```python
from build123d import *

# Parameters (mm, degrees)
FILLET1_R          = 1
FILLET2_R          = 3
CHAMFER1_SIZE      = 1
CUT_EXTRUDE2_START = 10
CUT_EXTRUDE2_DEPTH = 2
CHAMFER2_SIZE      = 1


with BuildPart() as part:
    # Sketch1 → Revolve1 (revolve)
    with BuildSketch(Plane(origin=(0, 0, 0), x_dir=(0, 0, -1), z_dir=(1, 0, 0))):
        with BuildLine():
            Line((0, 0), (0, -10))
            Line((0, -10), (-16.5, -10))
            Line((-16.5, -10), (-16.5, -15))
            Line((-16.5, -15), (-21.5, -15))
            Line((-21.5, -15), (-21.5, -12.5))
            ThreePointArc((-21.5, -12.5), (-22, -12), (-22.5, -12.5))
            Line((-22.5, -12.5), (-130, -12.5))
            Line((-130, -12.5), (-130, -10))
            Line((-130, -10), (-200, -10))
            Line((-200, -10), (-200, 0))
            Line((-200, 0), (0, 0))
        make_face()
    revolve(axis=Axis((0, 0, 0), (0, 0, 1)))

    # Fillet1
    fillet1_edges = [part.edges().sort_by_distance(p)[0] for p in [
        (0, 10, 130),
    ]]
    fillet(fillet1_edges, radius=FILLET1_R)

    # Fillet2
    fillet2_edges = [part.edges().sort_by_distance(p)[0] for p in [
        (0, 10, 16.5),
    ]]
    fillet(fillet2_edges, radius=FILLET2_R)

    # Chamfer1
    chamfer1_edges = [part.edges().sort_by_distance(p)[0] for p in [
        (0, 10, 200),
    ]]
    chamfer(chamfer1_edges, length=CHAMFER1_SIZE)

    # Sketch2 → Cut-Extrude2 (cut)
    with BuildSketch(Plane(origin=(0, 0, 0), x_dir=(0, 0, -1), z_dir=(1, 0, 0)).offset(CUT_EXTRUDE2_START)):
        with BuildLine():
            Line((-148, -2), (-152, -2))
            ThreePointArc((-152, -2), (-154, 0), (-152, 2))
            Line((-152, 2), (-148, 2))
            ThreePointArc((-148, 2), (-146, 0), (-148, -2))
        make_face()
    extrude(amount=-CUT_EXTRUDE2_DEPTH, mode=Mode.SUBTRACT)

    # Chamfer2
    chamfer2_edges = [part.edges().sort_by_distance(p)[0] for p in [
        (0, 10, 0),
    ]]
    chamfer(chamfer2_edges, length=CHAMFER2_SIZE)


solid = part.part
```
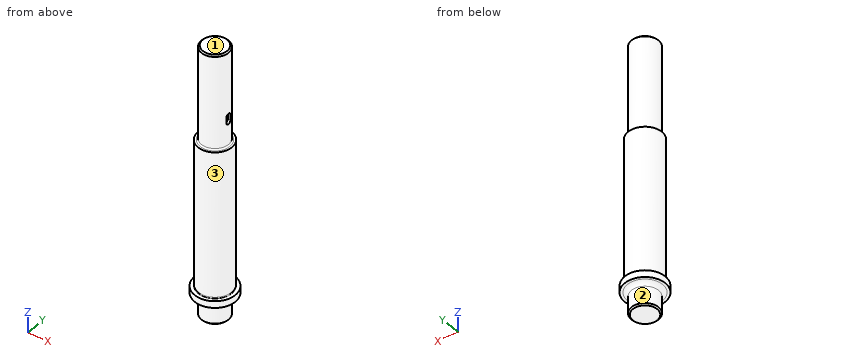
Model file for the job. Use its own axes, mm. Face numbers are marked on the shaded views. A direction names the side the tool comes from. Give positions to 0.01 mm unless a question says otherwise; leave off trailing zeros. Loops run counter-clockwise (first coordinate to the right, second up) from the corner with the lowest first, then second, coordinate; pieces in that order, holes last. Notation, with made-up numbers: (74.5, 38.25) -> (121.5, 38.25) arc R27 cw to (121.5, 75.25) -> close; hole circle Ø9 at (-6, 83). An arc over 180 degrees is marked (long way). Use CSV: the item, a comma, the result in double quotes. Start each with the question number.
1) Tool access for the marked faces 1, 2 and 3: list every direction of +Z, -Z, +X, -X, +Y, -Y with a clear straight run to the whole face (end or side of a thin tool).
2) Slice it at C-C on z = 100.5. Give the cut face in (x, y).
3) Flat gauge pins, fed straight in: pin 1 Ø5 at (x, z) = (10, 144) entering from +Y; pin 2 Ø2 at (y, z) = (0, 151) entering from +X; pin 3 Ø5 at (x, z) = (-11, 25.5) entering from +Y. Where does each tip first touch, or does it go through?
4) Wall check: line 1 (Z direction, x = 7.75, y = 11.25); line 2 (Y direction, x = -0.5, z = 109.5); line 3 (Y direction, x = 2, z = 182). Give the ranges that are in metal, low to high.
5) Slice it at B-B on z = 142. Give the cut face in (x, y).
Computed values:
1,face 1,"+Z, +X, -X, +Y, -Y"
1,face 2,"-Z"
1,face 3,"+Z"
2,outline,"circle Ø25 at (0, 0)"
3,pin 1,"stops at y = 6.61"
3,pin 2,"stops at x = 8"
3,pin 3,"stops at y = 9.17"
4,line 1,"z = 16.5 to 21.5"
4,line 2,"y = -12.49 to 12.49"
4,line 3,"y = -9.8 to 9.8"
5,outline,"circle Ø20 at (0, 0)"
